Can you work these out from the drawing? Everything is in mm from the part's minimum corner. Coordinates: 2 decimals unless noted, no trailing zeros. Loops run counter-clockwise (first coordinate to the right, second up) from the corner with the lowest first, then second, coordinate; pieces in that order, holes last. Notation, with made-up numbers: (47, -35) - (66, -35) arc R25 cw to (66, 4) - close; hole circle Ø5 at (0.25, 85.25). An arc over 180 degrees is marked (long way). Put each result on its own line as item: value. Start each with the question number.
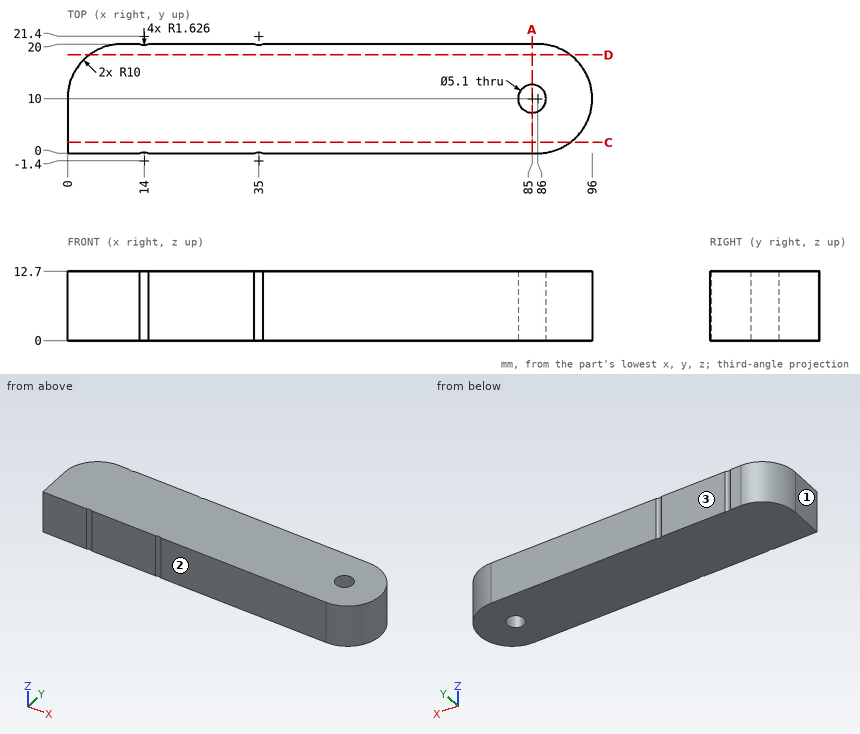
(1) I want a section at C-C on y = 2. List the corners of the cut face in (x, z) for me.
(2) I want a section at D-D on y = 18. List the corners of the cut face in (x, z) for me.
(3) I need wall thicknesses on L1, parallel to Y at x = 85, z = 7; L2, parallel to Y at x = 91, z = 7.25; L3, parallel to X at y = 7, z = 5.5. Which ranges of each line are inside material? Lowest first, please. Write a range as [from, to].
(4) If we mould it in two halves opening along Y, with no side actions, what happens to the marked faces 1, 2 and 3? For each: pulls with the +Y half, pulls with the -Y half, needs draft (parallel to the pull), parting line crosses it, or undercut.
(5) I want a section at A-A on x = 85. List the corners of the cut face in (y, z) for me.
(6) For pin 1 Ø8 at (x, y) = (85, 10) entering from -Z; pin 2 Ø6 at (y, z) = (15.5, 1.5) entering from -X, each with a flat end and sliding along its axis, tell me the tip position at first contact or that it passes through.
Answer sheet:
1. outline: (0, 0) - (92, 0) - (92, 12.7) - (0, 12.7) - close
2. outline: (4, 0) - (92, 0) - (92, 12.7) - (4, 12.7) - close
3. L1: y = [0, 7.45], [12.55, 20]
3. L2: y = [1.34, 18.66]
3. L3: x = [0, 95.54]
4. face 1: needs draft
4. face 2: pulls with the -Y half
4. face 3: pulls with the +Y half
5. outline: (0, 0) - (7.45, 0) - (7.45, 12.7) - (0, 12.7) - close; (12.55, 0) - (20, 0) - (20, 12.7) - (12.55, 12.7) - close
6. pin 1: stops at z = 0
6. pin 2: stops at x = 0.32
